Geometry: final body of the model. Coordinates: model frame, mm. A direction names the side the tool comes from. Give positions to 0.01 mm unless a question says otherwise; leave off trailing zeros. Loops run counter-clockwise (first coordinate to the right, second up) from the corner with the lowest first, then second, coordinate; pieces in that order, holes last. Notation, with made-up numbers: (1.5, -39.5) -> (59.5, -39.5) arc R29 cw to (59.5, -2.5) -> close; hole circle Ø5 at (65.25, 62). An arc over 180 degrees is marked (long way). One line per item, written item: value. Start each with the question number.
from build123d import *

# Parameters (mm, degrees)
SKETCH1_W           = 284.1625
SKETCH1_H           = 101.6
BOSS_EXTRUDE1_DEPTH = 73.025
SKETCH2_R           = 19.05
SKETCH2_R_2         = 4.7625
SKETCH2_R_3         = 3.96875
CUT_EXTRUDE1_DEPTH  = 168.631656397
SKETCH2_3_R         = 22.225
SKETCH2_3_R_2       = 6.35
CUT_EXTRUDE2_DEPTH  = 12.7
CUT_EXTRUDE3_START  = -31.75
SKETCH3_W           = 123.825
SKETCH3_H           = 38.1
SKETCH3_R           = 4.7625
CUT_EXTRUDE3_DEPTH  = 31.75
SKETCH3_3_W         = 19.05
SKETCH3_3_H         = 6.35
CUT_EXTRUDE4_DEPTH  = 168.631656397


with BuildPart() as part:
    # Sketch1 → Boss-Extrude1 (new body)
    with BuildSketch(Plane.XY):
        Rectangle(SKETCH1_W, SKETCH1_H)
    extrude(amount=BOSS_EXTRUDE1_DEPTH)

    # Sketch2 → Cut-Extrude1 (cut, through all)
    with BuildSketch(Plane.XY.offset(73.025)):
        with BuildLine():
            Line((111.91875, 4.7625), (107.15625, 4.7625))
            ThreePointArc((107.15625, 4.7625), (102.39375, 0), (107.15625, -4.7625))
            Line((107.15625, -4.7625), (111.91875, -4.7625))
            ThreePointArc((111.91875, -4.7625), (116.68125, 0), (111.91875, 4.7625))
        make_face()
        with Locations((-42.06875, -19.05)):
            Circle(SKETCH2_R)
        with Locations((34.13125, 0)):
            Circle(SKETCH2_R_2)
        with Locations((-13.499467703, -38.276580456)):
            Circle(SKETCH2_R_3)
        with Locations((-70.638032297, 0.176580456)):
            Circle(SKETCH2_R_3)
    extrude(amount=-CUT_EXTRUDE1_DEPTH, mode=Mode.SUBTRACT)

    # Sketch2_3 → Cut-Extrude2 (cut)
    with BuildSketch(Plane.XY.offset(73.025)):
        with Locations((-42.06875, -19.05)):
            Circle(SKETCH2_3_R)
        with Locations((34.13125, 0)):
            Circle(SKETCH2_3_R_2)
    extrude(amount=-CUT_EXTRUDE2_DEPTH, mode=Mode.SUBTRACT)

    # Sketch3 → Cut-Extrude3 (cut)
    with BuildSketch(Plane(origin=(0, 0, 0), x_dir=(-1, 0, 0), z_dir=(0, 0, -1)).offset(CUT_EXTRUDE3_START)):
        with Locations((-61.11875, 0)):
            Rectangle(SKETCH3_W, SKETCH3_H)
        with Locations(Location((-34.13125, 0, 0), (0, 0, 180))):
            Circle(SKETCH3_R, mode=Mode.SUBTRACT)
        with BuildLine():
            ThreePointArc((-107.15625, 4.7625), (-102.39375, 0), (-107.15625, -4.7625))
            Line((-107.15625, -4.7625), (-111.91875, -4.7625))
            ThreePointArc((-111.91875, -4.7625), (-116.68125, 0), (-111.91875, 4.7625))
            Line((-111.91875, 4.7625), (-107.15625, 4.7625))
        make_face(mode=Mode.SUBTRACT)
    extrude(amount=CUT_EXTRUDE3_DEPTH, mode=Mode.SUBTRACT)

    # Sketch3_3 → Cut-Extrude4 (cut, through all)
    with BuildSketch(Plane(origin=(0, 0, 0), x_dir=(-1, 0, 0), z_dir=(0, 0, -1))):
        with Locations((-8.73125, -47.625)):
            Rectangle(SKETCH3_3_W, SKETCH3_3_H)
        with Locations((113.50625, -47.625)):
            Rectangle(SKETCH3_3_W, SKETCH3_3_H)
    extrude(amount=-CUT_EXTRUDE4_DEPTH, mode=Mode.SUBTRACT)


solid = part.part
Item 1: Section B-B, the plane y = -23.5. Output: boundary loops of the cut face in (x, z) (3 decimals), then the cut area to 3 significant figures.
Item 2: Mould query, pull axis Y, two halves, no side actions, for faces 4 (the face through (-24, -12, 60.325)), 5 (the face through (-0.794, 0, 16)), 6 (the face through (79, -50.8, 36)), 7 (the face through (18.256, -48, 36)). Classes: pulls with the +Y half, pulls with the -Y half, needs draft (parallel to the pull), parting line crosses it, or undercut.
Item 3: Section C-C, the plane z = 22. Output: boundary loops of the cut face in (x, y), then the cut area to 3 significant figures.
Item 4: Pin query (flat end, axial travel): pin 1 (10 mm diameter, centred on x = 35, y = 0, fed in from +Z) (3 decimals); pin 2 (15 mm diameter, centred on x = -118, z = 48, fed in from -Y); pin 3 (19 mm diameter, centred on x = 35, y = 6, fed in from -Z). Return the tip coordinate at first contact, or that it passes through.
Item 5: Access query for faces 1 (the face through (-103.981, -48, 36)), 2 (the face through (116.68, -0.1, 52.68)), 3 (the face through (62, 0, 31.75)). Directions: +Z, -Z, +X, -X, +Y, -Y. A direction counts if a zero-diameter tool reaches every point of the face in a straight line with its end or side. Return the directions, or none.
Item 6: Section A-A, the plane x = -45. Output: boundary loops of the cut face in (y, z) (3 decimals), then the cut area to 3 significant figures.
Item 7: Ray query, line 1 along X through (y, z) = (-45, 24); line 2 along Y through (x, z) = (61, 10.5); line 3 along Z through (x, y) = (23, -2.5) (3 decimals). Return the intervals inside material, ascending. Write a range as [from, to].
Item 8: Section D-D, the plane x = 91. Output: boundary loops of the cut face in (y, z) (3 decimals), then the cut area to 3 significant figures.
Geometry check:
1. outline: (-142.081, 0) -> (-60.592, 0) -> (-60.592, 60.325) -> (-63.844, 60.325) -> (-63.844, 73.025) -> (-142.081, 73.025) -> close; (-23.546, 0) -> (142.081, 0) -> (142.081, 73.025) -> (-20.294, 73.025) -> (-20.294, 60.325) -> (-23.546, 60.325) -> close
1. area: 18,000 mm2
2. face 4: undercut
2. face 5: undercut
2. face 6: pulls with the -Y half
2. face 7: needs draft
3. outline: (-142.08, -50.8) -> (-123.03, -50.8) -> (-123.03, -44.45) -> (-103.98, -44.45) -> (-103.98, -50.8) -> (-0.79, -50.8) -> (-0.79, -44.45) -> (18.26, -44.45) -> (18.26, -50.8) -> (142.08, -50.8) -> (142.08, 50.8) -> (-142.08, 50.8) -> close; hole circle Ø7.94 at (-70.64, 0.18); hole circle Ø38.1 at (-42.07, -19.05); hole circle Ø7.94 at (-13.5, -38.28); hole (-0.79, -19.05) -> (123.03, -19.05) -> (123.03, 19.05) -> (-0.79, 19.05) -> close
3. area: 22,700 mm2
4. pin 1: stops at z = 60.325
4. pin 2: stops at y = -50.8
4. pin 3: stops at z = 31.75
5. face 1: +Z, -Z, -Y
5. face 2: +Z, -Z
5. face 3: -Z
6. outline: (-50.8, 0) -> (-37.873, 0) -> (-37.873, 60.325) -> (-41.081, 60.325) -> (-41.081, 73.025) -> (-50.8, 73.025) -> close; (-0.227, 0) -> (50.8, 0) -> (50.8, 73.025) -> (2.981, 73.025) -> (2.981, 60.325) -> (-0.227, 60.325) -> close
6. area: 4,590 mm2
7. line 1: x = [-142.08, -123.03], [-103.98, -0.79], [18.26, 142.08]
7. line 2: y = [-50.8, -19.05], [19.05, 50.8]
7. line 3: z = [31.75, 73.025]
8. outline: (-50.8, 0) -> (-19.05, 0) -> (-19.05, 31.75) -> (19.05, 31.75) -> (19.05, 0) -> (50.8, 0) -> (50.8, 73.025) -> (-50.8, 73.025) -> close
8. area: 6,210 mm2
